Design review of the part built by this model. Coordinates are the model's own, in mm. Face numbers are marked on the shaded views. A direction names the side the tool comes from. Round coordinates to 2 decimals unless told otherwise and drop trailing zeros. Order: outer loops, then holes, each group sorted by start corner. A loop starts at its lowest first (then second) coordinate and runs counter-clockwise, first axis right, second up. Notation, with made-up numbers: (25.5, -37.5) - (50.5, -37.5) arc R21 ccw to (50.5, -30.5) - close; hole circle Ø1 at (37.5, 82.25). An arc over 180 degrees is marked (long way). Use CSV: the item, a comma, the result in double quotes.
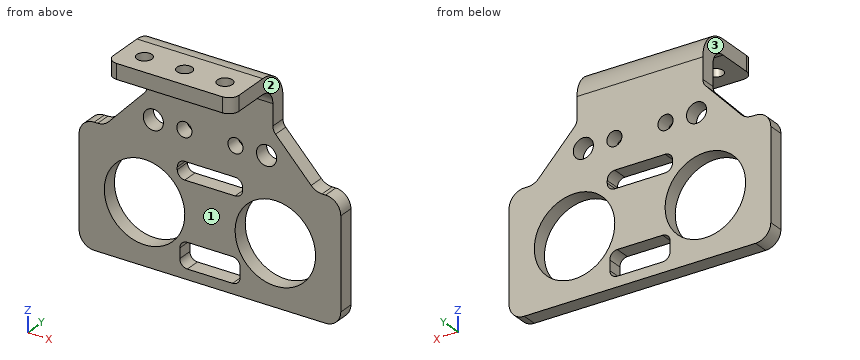
from build123d import *

# Parameters (mm, degrees)
CROQUIS11_R             = 2
CROQUIS11_R_2           = 1.5
CROQUIS11_R_3           = 9
SALIENTE_EXTRUIR1_DEPTH = 3
REDONDEO1_R             = 3
BOSS_EXTRUDE1_START     = -3
SKETCH1_R               = 9
SKETCH1_R_2             = 8
BOSS_EXTRUDE1_DEPTH     = 3
SKETCH2_W               = 25
SKETCH2_H               = 3
BOSS_EXTRUDE2_DEPTH     = 5
EDGE_FLANGE1_DEPTH      = 25
SKETCH10_R              = 1.5
CUT_EXTRUDE1_DEPTH      = 3
FILLET1_R               = 2


# Sheet-metal steps are written as plain solids
with BuildPart() as part:
    # Croquis11 → Saliente-Extruir1 (new body)
    with BuildSketch(Plane(origin=(0, 0, 0), x_dir=(1, 0, 0), z_dir=(0, 1, 0))):
        Polygon((-26, 18), (-21, 18), (-12.5, 9), (12.5, 9), (21, 18), (26, 18), (26, 42), (-26, 42), align=None)
        with Locations(Location((-11.25, 14.08, 0), (0, 0, 270))):
            Circle(CROQUIS11_R, mode=Mode.SUBTRACT)
        with Locations(Location((-5.08, 14.08, 0), (0, 0, 270))):
            Circle(CROQUIS11_R_2, mode=Mode.SUBTRACT)
        with Locations(Location((5.08, 14.08, 0), (0, 0, 90))):
            Circle(CROQUIS11_R_2, mode=Mode.SUBTRACT)
        with Locations(Location((11.25, 14.08, 0), (0, 0, 90))):
            Circle(CROQUIS11_R, mode=Mode.SUBTRACT)
        with Locations(Location((13, 30, 0), (0, 0, 270))):
            Circle(CROQUIS11_R_3, mode=Mode.SUBTRACT)
        with Locations(Location((-13, 30, 0), (0, 0, 270))):
            Circle(CROQUIS11_R_3, mode=Mode.SUBTRACT)
        with BuildLine():
            Line((-6, 38.5), (-6, 36.5))
            ThreePointArc((-6, 36.5), (-5.560660172, 35.439339828), (-4.5, 35))
            Line((-4.5, 35), (4.5, 35))
            ThreePointArc((4.5, 35), (5.560660172, 35.439339828), (6, 36.5))
            Line((6, 36.5), (6, 38.5))
            ThreePointArc((6, 38.5), (5.560660172, 39.560660172), (4.5, 40))
            Line((4.5, 40), (-4.5, 40))
            ThreePointArc((-4.5, 40), (-5.560660172, 39.560660172), (-6, 38.5))
        make_face(mode=Mode.SUBTRACT)
        with BuildLine():
            Line((6.5, 22), (6.5, 21.5))
            ThreePointArc((6.5, 21.5), (6.060660172, 20.439339828), (5, 20))
            Line((5, 20), (-5, 20))
            ThreePointArc((-5, 20), (-6.060660172, 20.439339828), (-6.5, 21.5))
            Line((-6.5, 21.5), (-6.5, 22))
            ThreePointArc((-6.5, 22), (-6.060660172, 23.060660172), (-5, 23.5))
            Line((-5, 23.5), (5, 23.5))
            ThreePointArc((5, 23.5), (6.060660172, 23.060660172), (6.5, 22))
        make_face(mode=Mode.SUBTRACT)
    extrude(amount=SALIENTE_EXTRUIR1_DEPTH)

    # Redondeo1
    redondeo1_edges = [part.edges().sort_by_distance(p)[0] for p in [
        (26, 1.5, -18),
        (21, 1.5, -18),
        (-21, 1.5, -18),
        (-26, 1.5, -18),
        (-26, 1.5, -42),
        (26, 1.5, -42),
    ]]
    fillet(redondeo1_edges, radius=REDONDEO1_R)

    # Sketch1 → Boss-Extrude1 (add)
    # profile 1 of 2: a face of its own
    with BuildSketch(Plane(origin=(0, 3, 0), x_dir=(1, 0, 0), z_dir=(0, 1, 0)).offset(BOSS_EXTRUDE1_START)):
        with Locations((-13, 30)):
            Circle(SKETCH1_R)
        with Locations(Location((-13, 30, 0), (0, 0, 270))):
            Circle(SKETCH1_R_2, mode=Mode.SUBTRACT)
    # profile 2 of 2: a face of its own
    with BuildSketch(Plane(origin=(0, 3, 0), x_dir=(1, 0, 0), z_dir=(0, 1, 0)).offset(BOSS_EXTRUDE1_START)):
        with Locations((13, 30)):
            Circle(SKETCH1_R)
        with Locations(Location((13, 30, 0), (0, 0, 270))):
            Circle(SKETCH1_R_2, mode=Mode.SUBTRACT)
    extrude(amount=BOSS_EXTRUDE1_DEPTH)

    # Sketch2 → Boss-Extrude2 (add)
    with BuildSketch(Plane.XY.offset(-9)):
        with Locations((0, 1.5)):
            Rectangle(SKETCH2_W, SKETCH2_H)
    extrude(amount=BOSS_EXTRUDE2_DEPTH)

    # Edge-Flange1 section (across the edge) → Edge-Flange1 (add)
    with BuildSketch(Plane(origin=(12.5, 0, -1), x_dir=(0, 0, -1), z_dir=(-1, 0, 0))):
        with BuildLine():
            Line((-3, 3), (-3, 12))
            Line((-3, 12), (0, 12))
            Line((0, 12), (0, 3))
            ThreePointArc((0, 3), (0.878679656, 0.878679656), (3, 0))
            Line((3, 0), (3, -3))
            ThreePointArc((3, -3), (-1.242640687, -1.242640687), (-3, 3))
        make_face()
    extrude(amount=EDGE_FLANGE1_DEPTH)

    # Sketch10 → Cut-Extrude1 (cut)
    with BuildSketch(Plane.XY.offset(2)):
        with Locations((0, -7.5)):
            Circle(SKETCH10_R)
        with Locations((-8, -7.5)):
            Circle(SKETCH10_R)
        with Locations((8, -7.5)):
            Circle(SKETCH10_R)
    extrude(amount=-CUT_EXTRUDE1_DEPTH, mode=Mode.SUBTRACT)

    # Fillet1
    fillet1_edges = [part.edges().sort_by_distance(p)[0] for p in [
        (12.5, 1.5, -9),
        (-12.5, 1.5, -9),
        (12.5, -12, 0.5),
        (-12.5, -12, 0.5),
    ]]
    fillet(fillet1_edges, radius=FILLET1_R)


solid = part.part
1) We need section A-A (y = -7.5). Give the boundary of the cut face in (x, z), then the cut area to 3 significant figures.
Data:
outline,"(-12.5, -1) - (-9.5, -1) - (-9.5, 2) - (-12.5, 2) - close; (-6.5, -1) - (-1.5, -1) - (-1.5, 2) - (-6.5, 2) - close; (1.5, -1) - (6.5, -1) - (6.5, 2) - (1.5, 2) - close; (9.5, -1) - (12.5, -1) - (12.5, 2) - (9.5, 2) - close"
area,"48.0 mm2"
2) For the marked faces 1, 2 and 3, list the 3-axis set-ups (+Z, -Z, +X, -X, +Y, -Y) from which the entire face can be reached by the end or side of a thin tool; tool diameter is ignored.
Data:
face 1,"-Z, +X, -X, -Y"
face 2,"+Z, +X, +Y, -Y"
face 3,"+Z, -X, +Y, -Y"
3) Insertion check: pin 1 Ø2 at (x, y) = (-12.5, -4) entering from -Z; pin 2 Ø6 at (y, z) = (-8, -3.5) entering from +X; pin 3 Ø3.5 at (x, y) = (0.5, 1) entering from +Z; pin 4 Ø6.5 at (x, z) = (11.25, -14.08) entering from +Y. Each pin has a flat end and moves straight along its axis. Give the tip position at first contact, or say it passes through.
Data:
pin 1,"stops at z = -1"
pin 2,"stops at x = 12.5"
pin 3,"stops at z = 1.56"
pin 4,"stops at y = 3"
4) We need section C-C (x = 0). Give the boundary of the cut face in (y, z).
Data:
outline,"(-12, -1) - (-9, -1) - (-9, 2) - (-12, 2) - close; (-6, -1) - (-3, -1) arc R3 cw to (0, -4) - (0, -20) - (3, -20) - (3, -4) arc R6 ccw to (-3, 2) - (-6, 2) - close; (0, -42) - (3, -42) - (3, -40) - (0, -40) - close; (0, -35) - (3, -35) - (3, -23.5) - (0, -23.5) - close"
5) To check wall thickness, follow L1, parallel to X at y = 2.1, z = -30; L2, parallel to Z at x = -11, y = 2; L3, parallel to X at y = -8, z = 0.5. State the ranges of each line that lie inside material, in increasing order. Write a range as from..to.
Data:
L1,"x = -26..-21, -5..5, 21..26"
L2,"z = -42..-37.75, -22.25..-16.06, -12.1..-0.68"
L3,"x = -12.5..-9.41, -6.59..-1.41, 1.41..6.59, 9.41..12.5"
6) We need section D-D (x = 8). Give the boundary of the cut face in (y, z) (3 decimals).
Data:
outline,"(-12, -1) - (-9, -1) - (-9, 2) - (-12, 2) - close; (-6, -1) - (-3, -1) arc R3 cw to (0, -4) - (0, -23.755) - (3, -23.755) - (3, -4) arc R6 ccw to (-3, 2) - (-6, 2) - close; (0, -42) - (3, -42) - (3, -36.245) - (0, -36.245) - close"
7) We need section B-B (x = 16). Give the boundary of the cut face in (y, z), then the cut area to 3 significant figures.
Data:
outline,"(0, -42) - (3, -42) - (3, -37.42) - (0, -37.42) - close; (0, -22.58) - (3, -22.58) - (3, -12.71) - (0, -12.71) - close"
area,"43.4 mm2"
